Build history of the part. All positions in model axes, mm. A direction names the side the tool comes from. Give positions to 0.01 mm unless a question says otherwise; leave off trailing zeros. Loops run counter-clockwise (first coordinate to the right, second up) from the corner with the lowest first, then second, coordinate; pieces in that order, holes last. Notation, with made-up numbers: (89, 0) -> (146, 0) arc R16 cw to (146, 19) -> close; hole circle Ø11 at (-24, 10). An arc over 180 degrees is marked (long way). Answer as a JSON object with one key per item and string values. Group by question number.
Q1. Drop flat-ended pins along their axis: pin 1 (3.5 mm diameter, centred on x = 15, z = 0, fed in from -Y); pin 2 (1.5 mm diameter, centred on y = 9, z = 2, fed in from -X). Give the stop position or say it passes through.
Q2. Wall check: probe 1 along Y at (x, z) = (-10.5, 2); probe 2 along Z at (x, y) = (15, 15); probe 3 along X at (y, z) = (24.5, -1). Give the ranges that are in metal, low to high. Write a range as from..to.
Q3. Band-saw the part on A-A, the plane y = 8. Write the cut outline in (x, z), plus the area to 3 significant figures.
Q4. Band-saw the part on C-C, the plane y = 23. Write the cut outline in (x, z), plus the area to 3 significant figures.
Q5. Tool access for faces 1 (the cylindrical face through (8.422, 9.806, -0.056)), 2 (the flat face through (19, 17, 0)): list every direction of +Z, -Z, +X, -X, +Y, -Y with a clear straight run to the whole face (end or side of a thin tool).
Q6. Band-saw the part on D-D, the plane z = -2.75. Write the cut outline in (x, y), plus the area to 3 significant figures.
Q7. Two-plate mould, pull along Z, no slides. Class faces 3 (the cylindrical face through (-18, 17.74, 2.95)), 4 (the flat face through (12.5, 12, 0)), 5 (the cylindrical face through (16.9, 17.26, -0.08)): pulls with the +Z half, pulls with the -Z half, needs draft (parallel to the pull), parting line crosses it, or undercut.
Q8. Band-saw the part on B-B, the plane x = -7.5. Write the cut outline in (y, z).
Autodesk Inventor part; units mm, degrees
ref_plane "YZ Plane" through (0, 0, 0) normal (1, 0, 0) x (0, 1, 0)
ref_plane "XZ Plane" through (0, 0, 0) normal (0, 1, 0) x (-1, 0, 0)
ref_plane "XY Plane" through (0, 0, 0) normal (0, 0, 1) x (1, 0, 0)
sketch "Эскиз1" plane through (0, 0, 0) normal (1, 0, 0) x (0, 1, 0)
  point P0 (0, 0)
sketch "Эскиз2" plane through (0, 0, 0) normal (0, 1, 0) x (-1, 0, 0)
  line L0 (19, -4) -> (-19, -4)
  line L1 (-19, -4) -> (-19, 4)
  line L2 (-19, 4) -> (19, 4)
  line L3 (19, 4) -> (19, -4)
  line L4 (19, -4) -> (-19, 4) construction
  line L5 (-19, -4) -> (19, 4) construction
  line L6 (19, 0) -> (-19, 0) construction
  circle A0 centre (-15, 0) radius 1.9
  line L7 (0, -4) -> (0, 4) construction
  circle A1 centre (15, 0) radius 1.9
  point P0 (0, 0)
  dimension "d1" = 30
  dimension "d2" = 3.8
  dimension "d3" = 38
  dimension "d4" = 8
extrude "Выдавливание1" add sketch "Эскиз2" along normal blind 35
fillet "Сопряжение1" radius 3.5 4 edges at (19, 17.5, 4) (19, 17.5, -4) (-19, 17.5, 4) (-19, 17.5, -4)
sketch "Эскиз3" plane through (-15.5, 0, 4) normal (0, 0, 1) x (1, 0, 0)
  line L0 (28.6, 35) -> (28.6, 0) construction
  line L1 (0, 0) -> (0, 35) construction
  line L2 (0, 0) -> (31, 0) construction
  line L3 (31, 35) -> (31, 0) construction
  line L4 (0, 35) -> (31, 35) construction
  line L5 (32.4, 35) -> (32.4, 0) construction
  line L6 (34.5, 35) -> (31, 35) construction
  line L7 (31, 35) -> (31, 0) construction
  line L8 (31, 0) -> (34.5, 0) construction
  line L9 (34.5, 0) -> (34.5, 35) construction
  line L10 (-1.4, 35) -> (-1.4, 0) construction
  line L11 (0, 35) -> (-3.5, 35) construction
  line L12 (-3.5, 35) -> (-3.5, 0) construction
  line L13 (-3.5, 0) -> (0, 0) construction
  line L14 (0, 0) -> (0, 35) construction
  line L15 (0, 0) -> (0, 35) construction
  line L16 (-1.4, 35) -> (2.4, 35) construction
  line L17 (28.6, 35) -> (32.4, 35) construction
  line L18 (28.6, 0) -> (32.4, 0) construction
  line L19 (-1.4, 35) -> (2.4, 35) construction
  line L20 (-1.4, 0) -> (2.4, 0) construction
  line L21 (-1.4, 35) -> (2.4, 35) construction
  line L22 (-1.4, 0) -> (2.4, 0) construction
  line L23 (2.4, 35) -> (2.4, 0) construction
  line L24 (28.6, 35) -> (2.4, 0) construction
  line L25 (2.4, 35) -> (28.6, 0) construction
  line L26 (15.5, 17.5) -> (15.5, 35) construction
  line L27 (0, 35) -> (31, 35) construction
  circle A0 centre (15.5, 12) radius 8.5
  point P0 (15.5, 0)
  dimension "d8" = 17
  dimension "d9" = 12
extrude "Выдавливание2" cut sketch "Эскиз3" against normal blind 35
sketch "Эскиз4" plane through (-15.5, 0, 4) normal (0, 0, 1) x (1, 0, 0)
  circle A0 centre (15.5, 12) radius 8.5
  line L0 (0, 0) -> (0, 35) construction
  line L1 (0, 0) -> (31, 0) construction
  line L2 (31, 35) -> (31, 0) construction
  line L3 (0, 35) -> (31, 35) construction
  line L4 (23.7614, 14) -> (28, 14)
  line L5 (28, 14) -> (28, 10)
  line L6 (28, 10) -> (23.7614, 10)
  line L7 (24, 10) -> (24, 14) construction
  circle A1 centre (15.5, 12) radius 8.5 construction
  line L8 (7, 12) -> (24, 12) construction
  line L9 (15.5, 12) -> (15.5, 20.5) construction
  line L10 (7.2386, 14) -> (3, 14)
  line L11 (3, 14) -> (3, 10)
  line L12 (3, 10) -> (7.2386, 10)
  point P0 (15.5, 0)
  dimension "d13" = 4
  dimension "d14" = 4
extrude "Выдавливание3" cut sketch "Эскиз4" against normal blind 10 contours A0 L4 L5 L6 | A0 L12 L11 L10
fillet "Сопряжение2" radius 1 8 edges at (-12.5, 14, 0) (-12.5, 10, 0) (-8.2614, 14, 0) (-8.2614, 10, 0) (8.2614, 14, 0) (8.2614, 10, 0) (12.5, 10, 0) (12.5, 14, 0)
properties part number "inner_mount" material "Пластик АБС"
Worked answers:
{
 "1": {"pin 1": "through", "pin 2": "x = -18.92"},
 "2": {"probe 1": "0..10, 14..35", "probe 2": "-4..-1.9, 1.9..4", "probe 3": "-18.96..-16.62, -13.38..13.38, 16.62..18.96"},
 "3": {"outline": "(-19, -0.5) arc R3.5 ccw to (-15.5, -4) -> (-7.5, -4) -> (-7.5, 4) -> (-15.5, 4) arc R3.5 ccw to (-19, 0.5) -> close; (7.5, -4) -> (15.5, -4) arc R3.5 ccw to (19, -0.5) -> (19, 0.5) arc R3.5 ccw to (15.5, 4) -> (7.5, 4) -> close; hole circle Ø3.8 at (-15, 0); hole circle Ø3.8 at (15, 0)", "area": "151 mm2"},
 "4": {"outline": "(-19, -0.5) arc R3.5 ccw to (-15.5, -4) -> (15.5, -4) arc R3.5 ccw to (19, -0.5) -> (19, 0.5) arc R3.5 ccw to (15.5, 4) -> (-15.5, 4) arc R3.5 ccw to (-19, 0.5) -> close; hole circle Ø3.8 at (-15, 0); hole circle Ø3.8 at (15, 0)", "area": "271 mm2"},
 "5": {"face 1": "+Z, -Z", "face 2": "+Z, -Z, +X, +Y, -Y"},
 "6": {"outline": "(-18.18, 0) -> (18.18, 0) -> (18.18, 35) -> (-18.18, 35) -> close; hole (-12.5, 11) arc R1 ccw to (-11.5, 10) -> (-9.01, 10) arc R1 cw to (-8.07, 9.32) arc R8.5 ccw to (8.07, 9.32) arc R1 cw to (9.01, 10) -> (11.5, 10) arc R1 ccw to (12.5, 11) -> (12.5, 13) arc R1 ccw to (11.5, 14) -> (9.01, 14) arc R1 cw to (8.07, 14.68) arc R8.5 ccw to (-8.07, 14.68) arc R1 cw to (-9.01, 14) -> (-11.5, 14) arc R1 ccw to (-12.5, 13) -> close", "area": "1,010 mm2"},
 "7": {"face 3": "pulls with the +Z half", "face 4": "needs draft", "face 5": "undercut"},
 "8": {"outline": "(0, -4) -> (8, -4) -> (8, 4) -> (0, 4) -> close; (16, -4) -> (35, -4) -> (35, 4) -> (16, 4) -> close"}
}
